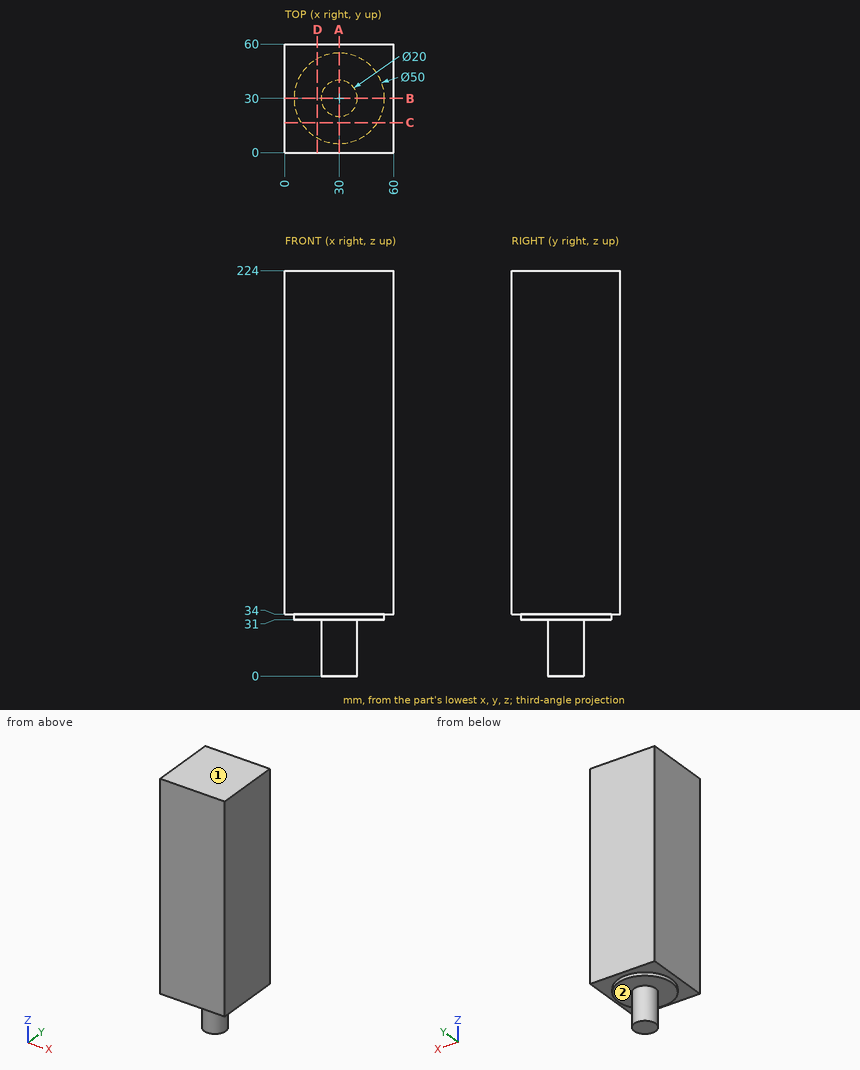
Print and shaded views of the part. All mm, measured from the part's lowest x, y and z. A direction names the side the tool comes from. Coordinates: 2 decimals unless noted, no trailing zeros. Write each loop counter-clockwise with the first axis right and the second up, starting at its lowest first coordinate (ties: lowest second). Pieces come first, ordered by that corner, then holes.
(1) Flat gauge pin, fed straight in: pin 1 (8 mm diameter, centred on x = 42, y = 7, fed in from -Z). Where does the tip first touch, or does it go through?
(2) Drill centre lines: probe 1 along Y at (x, z) = (29.5, 16); probe 2 along Z at (x, y) = (33, 17); probe 3 along Z at (x, y) = (54, 50.5). Where is each one in solid material? Low to high.
(3) Cut at A-A, the plane x = 30. List the corners of the cut face in (y, z).
(4) Cut at C-C, the plane y = 16.5. List the corners of the cut face in (x, z).
(5) 3-axis set-ups, long thin cutter, end or side, ignore diameter. For the marked faces 1 and 2: which of +Z, -Z, +X, -X, +Y, -Y reach the whole face in a straight line?
(6) Cut at D-D, the plane x = 18. List the corners of the cut face in (y, z), and give its area (3 significant figures).
Geometry says:
1. pin 1: stops at z = 31
2. probe 1: y = 20.01 to 39.99
2. probe 2: z = 31 to 224
2. probe 3: z = 34 to 224
3. outline: (0, 34) - (5, 34) - (5, 31) - (20, 31) - (20, 0) - (40, 0) - (40, 31) - (55, 31) - (55, 34) - (60, 34) - (60, 224) - (0, 224) - close
4. outline: (0, 34) - (8.96, 34) - (8.96, 31) - (51.04, 31) - (51.04, 34) - (60, 34) - (60, 224) - (0, 224) - close
5. face 1: +Z, +X, -X, +Y, -Y
5. face 2: -Z
6. outline: (0, 34) - (8.07, 34) - (8.07, 31) - (51.93, 31) - (51.93, 34) - (60, 34) - (60, 224) - (0, 224) - close
6. area: 11,500 mm2
